from build123d import *

# Parameters (mm, degrees)
F0_W     = 101.6
F0_H     = 101.6
F1_DEPTH = 101.6
F2_W     = 25.4
F2_H     = 25.4
F3_DEPTH = 101.6
F5_DEPTH = 101.6
F6_W     = 50.8
F6_H     = 25.4
F7_DEPTH = 101.6


with BuildPart() as f1:
    # F0 (on Front) → F1 (new body)
    with BuildSketch(Plane.XZ):
        with Locations((-103.523429, -35.627711)):
            Rectangle(F0_W, F0_H)
    extrude(amount=F1_DEPTH)

    # F2 (on face) → F3 (cut)
    with BuildSketch(Plane.XZ.offset(101.6)):
        with Locations((-65.423429, -22.927711)):
            Rectangle(F2_W, F2_H)
        with Locations((-141.623429, -22.927711)):
            Rectangle(F2_W, F2_H)
    extrude(amount=-F3_DEPTH, mode=Mode.SUBTRACT)

    # F4 (on face) → F5 (cut)
    with BuildSketch(Plane.XZ.offset(101.6)):
        Polygon((-128.923429, 15.172289), (-103.523429, -10.227711), (-78.123429, 15.172289), align=None)
    extrude(amount=-F5_DEPTH, mode=Mode.SUBTRACT)

    # F6 (on face) → F7 (cut)
    with BuildSketch(Plane.XZ.offset(101.6)):
        with Locations((-103.523429, -73.727711)):
            Rectangle(F6_W, F6_H)
    extrude(amount=-F7_DEPTH, mode=Mode.SUBTRACT)


solid = f1.part
Verification items for the finished model (mm, model axes). A direction names the side the tool comes from. Give positions to 0.01 mm unless a question says otherwise; leave off trailing zeros. Order: outer loops, then holes, each group sorted by start corner. A loop starts at its lowest first (then second) coordinate and runs counter-clockwise, first axis right, second up. Notation, with made-up numbers: M 31,-28.5 L 81,-28.5 A26 cw 81,4.5 Z; hole C 40,-31.5 d2. An arc over 180 degrees is marked long. Use one line per item in the form item = value. Start each with the question number.
Q1. Section check D-D (x = -127.5). Enter the section's corners in (y, z).
Q2. Mould release check, pull along Z, two halves, no side actions. Record for faces 5 (the flat face through (-142, -52, -35.628)), 6 (the flat face through (-104, 0, -35)), 7 (the flat face through (-142, -50, 15.172)): +Z half, -Z half, draft (parallel to the pull), parting line (faces both ways), or undercut.
Q3. Access from +Z, -Z, +X, -X, +Y, -Y to the whole of each face (thin tool, end or side, straight path). Record for faces 1 (the flat face through (-104, -52, -61.028)), 2 (the flat face through (-78.123, -52, -23)), 3 (the flat face through (-91.001, -51.511, 2.294)), 4 (the flat face through (-142, -52, -10.228)).
Q4. Section check B-B (z = -76). Enter the section's corners in (x, y), then the cut area to 3 significant figures.
Q5. Section check A-A (x = -76). Enter the section's corners in (y, z).
Q6. Go/stop test with flat-tipped pins: pin 1 Ø8 at (x, y) = (-87, -89.5) entering from +Z; pin 2 Ø1 at (x, z) = (-124, -19) entering from +Y; pin 3 Ø12.5 at (y, z) = (-71.5, -25.5) entering from +X; pin 4 Ø1 at (y, z) = (-33, -31.5) entering from -X. Record where each tip stops, or that it passes through.
Q7. Scan lines: line 1 along Z through (x, y) = (-66.5, -29.5); line 2 along X through (y, z) = (-62, -68); line 3 along X through (y, z) = (-87.5, -28.5). Record each from-to range of solid material in increasing order. Write a range as [from, to].
Q8. Section check C-C (y = -84). Enter the section's corners in (x, z), then the cut area to 3 significant figures.
Evaluation:
q1.outline = M -101.6,-61.03 L 0,-61.03 L 0,13.75 L -101.6,13.75 Z
q2.face_5 = undercut
q2.face_6 = draft
q2.face_7 = +Z half
q3.face_1 = -Z, +Y, -Y
q3.face_2 = +X, +Y, -Y
q3.face_3 = +Z, +Y, -Y
q3.face_4 = -X, +Y, -Y
q4.outline = M -154.32,-101.6 L -128.92,-101.6 L -128.92,0 L -154.32,0 Z; M -78.12,-101.6 L -52.72,-101.6 L -52.72,0 L -78.12,0 Z
q4.area = 5,160 mm2
q5.outline = M -101.6,-86.43 L 0,-86.43 L 0,-35.63 L -101.6,-35.63 Z; M -101.6,-10.23 L 0,-10.23 L 0,15.17 L -101.6,15.17 Z
q6.pin_1 = 10.3
q6.pin_2 = 0
q6.pin_3 = -78.12
q6.pin_4 = -128.92
q7.line_1 = [-86.43, -35.63], [-10.23, 15.17]
q7.line_2 = [-154.32, -128.92], [-78.12, -52.72]
q7.line_3 = [-128.92, -78.12]
q8.outline = M -154.32,-86.43 L -128.92,-86.43 L -128.92,-61.03 L -78.12,-61.03 L -78.12,-86.43 L -52.72,-86.43 L -52.72,-35.63 L -78.12,-35.63 L -78.12,-10.23 L -52.72,-10.23 L -52.72,15.17 L -78.12,15.17 L -103.52,-10.23 L -128.92,15.17 L -154.32,15.17 L -154.32,-10.23 L -128.92,-10.23 L -128.92,-35.63 L -154.32,-35.63 Z
q8.area = 7,100 mm2
